Autodesk Inventor part; units mm, degrees
ref_plane "YZ Plane" through (0, 0, 0) normal (1, 0, 0) x (0, 1, 0)
ref_plane "XZ Plane" through (0, 0, 0) normal (0, 1, 0) x (-1, 0, 0)
ref_plane "XY Plane" through (0, 0, 0) normal (0, 0, 1) x (1, 0, 0)
sketch "Sketch1" plane through (0, 0, 0) normal (0, 1, 0) x (-1, 0, 0)
  line L0 (0, 0) -> (0, -1300)
  line L1 (550, -750) -> (550, -550)
  line L2 (150, -150) -> (150, -230)
  line L3 (150, -230) -> (230, -230)
  line L4 (0, 0) -> (150, -150)
  line L5 (230, -230) -> (550, -550)
  line L6 (150, -1150) -> (150, -1070)
  line L7 (150, -1070) -> (230, -1070)
  line L8 (0, -1300) -> (150, -1150)
  line L9 (230, -1070) -> (550, -750)
  dimension "d3" = 1300
  dimension "d6" = 550
  dimension "d7" = 150
  dimension "d8" = 80
  dimension "d9" = 45
  dimension "d10" = 80
  dimension "d11" = 150
  dimension "d12" = 45
extrude "Extrusion1" add sketch "Sketch1" along normal blind 20
fillet "Fillet1" radius 5 1 edges at (-150, 10, -230)
fillet "Fillet2" radius 5 1 edges at (-150, 10, -1070)
properties part number "top short"
Design review of the part built by this model. Coordinates are the model's own, in mm. Coordinates: 2 decimals unless noted, no trailing zeros. Order: outer loops, then holes, each group sorted by start corner. A loop starts at its lowest first (then second) coordinate and runs counter-clockwise, first axis right, second up.
Item 1: Take a section at A-A, the plane y = 16.75. Write out the cut boundary in (x, z), then the cut area to 3 significant figures.
Item 2: Take a section at B-B, the plane z = -256.5. Write out the cut boundary in (x, y), then the cut area to 3 significant figures.
Item 3: For pin 1 Ø1 at (y, z) = (6.5, -711.5) entering from +X; pin 2 Ø10 at (x, y) = (-185, 10) entering from +Z; pin 3 Ø10 at (x, y) = (-93, 3.5) entering from +Z; pin 4 Ø1 at (y, z) = (17, -759) entering from -X, all flat-tipped, find the tip position at first contact; note any pin that passes through.
Item 4: For line 1 (Z direction, x = -412.5, y = 9.5); line 2 (Z direction, x = -206, y = 13.75); line 3 (X direction, y = 16.75, z = -1057), list the stretches that pass through material, from the lowest coordinate up.
Item 5: Take a section at C-C, the plane x = -342.5. Write out the cut boundary in (y, z), then the cut area to 3 significant figures.
The answers:
1. outline: (-550, -750) - (-230, -1070) - (-155, -1070) arc R5 cw to (-150, -1075) - (-150, -1150) - (0, -1300) - (0, 0) - (-150, -150) - (-150, -225) arc R5 cw to (-155, -230) - (-230, -230) - (-550, -550) - close
1. area: 406,000 mm2
2. outline: (-256.5, 0) - (0, 0) - (0, 20) - (-256.5, 20) - close
2. area: 5,130 mm2
3. pin 1: stops at x = 0
3. pin 2: stops at z = -230
3. pin 3: stops at z = -88
3. pin 4: stops at x = -541.5
4. line 1: z = -887.5 to -412.5
4. line 2: z = -1070 to -230
4. line 3: x = -243 to 0
5. outline: (0, -957.5) - (20, -957.5) - (20, -342.5) - (0, -342.5) - close
5. area: 12,300 mm2
